Autodesk Inventor part; units mm, degrees
ref_plane "YZ Plane" through (0, 0, 0) normal (1, 0, 0) x (0, 1, 0)
ref_plane "XZ Plane" through (0, 0, 0) normal (0, 1, 0) x (-1, 0, 0)
ref_plane "XY Plane" through (0, 0, 0) normal (0, 0, 1) x (1, 0, 0)
sketch "Skizze1" plane through (0, 0, 0) normal (0, 1, 0) x (-1, 0, 0)
  circle A0 centre (0, 0) radius 31.25
  circle A1 centre (0, 0) radius 33
  line L0 (0, 109.2005) -> (0, -98.3382) construction
  line L1 (65.6021, 0) -> (-69.7309, 0) construction
  line L2 (-37.5074, 64.9647) -> (55.9703, -96.9435) construction
  line L3 (-38.0847, -65.9646) -> (43.9559, 76.1338) construction
  line L4 (30, 1.25) -> (87, 1.25)
  line L5 (87, 1.25) -> (87, -1.25)
  line L6 (87, -1.25) -> (30, -1.25)
  line L7 (30, -1.25) -> (30, 1.25)
  line L8 (28, -3.25) -> (89, -3.25)
  line L9 (89, -3.25) -> (89, 3.25)
  line L10 (89, 3.25) -> (28, 3.25)
  line L11 (28, 3.25) -> (28, -3.25)
  line L12 (-16.0825, 25.3558) -> (-44.5825, 74.7192)
  line L13 (-42.4175, 75.9692) -> (-13.9175, 26.6058)
  line L14 (-11.1854, 25.8737) -> (-41.6854, 78.7013)
  line L15 (-47.3146, 75.4513) -> (-16.8146, 22.6237)
  line L16 (-44.5825, 74.7192) -> (-42.4175, 75.9692)
  line L17 (-41.6854, 78.7013) -> (-47.3146, 75.4513)
  line L18 (-13.9175, 26.6058) -> (-16.0825, 25.3558)
  line L19 (-16.8146, 22.6237) -> (-11.1854, 25.8737)
  line L20 (-13.9175, -26.6058) -> (-42.4175, -75.9692)
  line L21 (-44.5825, -74.7192) -> (-16.0825, -25.3558)
  line L22 (-16.8146, -22.6237) -> (-47.3146, -75.4513)
  line L23 (-41.6854, -78.7013) -> (-11.1854, -25.8737)
  line L24 (-42.4175, -75.9692) -> (-44.5825, -74.7192)
  line L25 (-47.3146, -75.4513) -> (-41.6854, -78.7013)
  line L26 (-16.0825, -25.3558) -> (-13.9175, -26.6058)
  line L27 (-11.1854, -25.8737) -> (-16.8146, -22.6237)
  point P0 (-32.8011, 56.8131)
  point P1 (-32.8011, -56.8131)
  point P2 (32.8396, -3.25)
  point P3 (32.8396, 3.25)
  point P4 (-13.6052, 30.0649)
  point P5 (-19.2344, 26.8149)
  point P6 (-19.2344, -26.8149)
  point P7 (-13.6052, -30.0649)
  point P8 (31.225, -1.25)
  point P9 (-14.53, -27.6666)
  point P10 (-16.695, -26.4166)
  point P11 (-16.695, 26.4166)
  point P12 (-14.53, 27.6666)
  point P13 (31.225, 1.25)
  dimension "d0" = 62.5
  dimension "d1" = 66
  dimension "d2" = 120
  dimension "d3" = 120
  dimension "d4" = 2.5
  dimension "d5" = 2
  dimension "d6" = 57
  dimension "d7" = 30
  dimension "d10" = 360
extrude "Extrusion1" add sketch "Skizze1" along normal blind 10 contours A0 L10 A1 L4 | L6 A1 L8 A0 | A0 L14 A1 L10 | A1 L10 L9 L8 L6 L5 L4 | L8 A1 L23 A0 | A0 L13 A1 L14 | L23 A1 L20 A0 | A1 L13 L16 L12 L15 L17 L14 | L23 L25 L22 A1 L21 L24 L20 | A0 L15 A1 L12 | L21 A1 L22 A0 | A0 L22 A1 L15
fillet "Rundung1" radius 2 6 edges at (-31.225, 5, -1.25) (-31.225, 5, 1.25) (14.53, 5, 27.6666) (16.695, 5, 26.4166) (16.695, 5, -26.4166) (14.53, 5, -27.6666)
chamfer "Fase1" distance 1 angle 45 15 edges at (-15.625, 10, -27.0633) (14.3424, 10, -28.3783) (28.9402, 10, -52.6258) (-31.7475, 10, -1.7683) (-60.0454, 10, -1.25) (31.25, 10, 0) (17.4051, 10, 26.61) (31.1052, 10, 51.3758) (17.4051, 10, -26.61) (31.1052, 10, -51.3758) (-15.625, 10, 27.0633) (-31.7475, 10, 1.7683) (-60.0454, 10, 1.25) (14.3424, 10, 28.3783) (28.9402, 10, 52.6258)
sketch "Skizze2" plane through (0, 0, 0) normal (0, 1, 0) x (-1, 0, 0)
  line L0 (-47.3146, 75.4513) -> (-19.2344, 26.8149)
  line L1 (-38.5127, 60.2059) -> (-38.5127, -59.496)
  line L2 (-38.5127, -59.496) -> (-38.5127, -60.2059)
  line L3 (-19.2344, -26.8149) -> (-47.3146, -75.4513)
  line L4 (-42.8652, 67.7448) -> (-42.8652, -67.7448)
  line L5 (-42.8652, -59.496) -> (-42.8652, -60.2059)
  line L6 (-38.5127, 60.2059) -> (-42.8652, 67.7448)
  line L7 (-38.4567, -60.109) -> (-42.8652, -67.7448)
  line L8 (-32.8835, -63.4559) -> (70.7814, -3.605)
  line L9 (70.7814, -3.605) -> (71.3962, -3.25)
  line L10 (-37.2361, -70.9948) -> (80.1013, -3.25)
  line L11 (72.9577, -7.3744) -> (73.5725, -7.0194)
  line L12 (-32.8835, -63.4559) -> (-37.2361, -70.9948)
  line L13 (71.2843, -3.25) -> (80.1013, -3.25)
  line L14 (71.3962, 3.25) -> (-32.2687, 63.101)
  line L15 (-32.2687, 63.101) -> (-32.8835, 63.4559)
  line L16 (80.1013, 3.25) -> (-37.2361, 70.9948)
  line L17 (-30.0925, 66.8704) -> (-30.7073, 67.2254)
  line L18 (71.3962, 3.25) -> (80.1013, 3.25)
  line L19 (-32.8276, 63.359) -> (-37.2361, 70.9948)
  point P0 (0, 0)
  point P1 (-41.6854, -78.7013)
  point P2 (-13.6052, -30.0649)
  point P3 (32.8396, -3.25)
  point P4 (89, -3.25)
  point P5 (89, 3.25)
  point P6 (32.8396, 3.25)
  point P7 (-13.6052, 30.0649)
  point P8 (-41.6854, 78.7013)
  dimension "d20" = 360
extrude "Extrusion2" add sketch "Skizze2" along normal blind 10
properties part number "_3D-Druck"
Model file for the job. Use its own axes, mm. A direction names the side the tool comes from. Coordinates: 2 decimals unless noted, no trailing zeros. Loops run counter-clockwise (first coordinate to the right, second up) from the corner with the lowest first, then second, coordinate; pieces in that order, holes last. Notation, with made-up numbers: M -17.75,55 L 14.25,55 A19 cw 14.25,80 Z; hole C 39,-34.5 d5. An arc over 180 degrees is marked long. Use CSV: the item, a comma, the result in double quotes. Start each with the question number.
1. Band-saw the part on A-A, the plane z = 48. List the corners of the cut face in (x, y), then the cut area to 3 significant figures.
2. Band-saw the part on B-B, the plane x = -35. List the corners of the cut face in (y, z), then the cut area to 3 significant figures.
3. Two-plate mould, pull along X, no slides. Class faces 5 (the flat face through (-85, 5, 3.25)), 6 (the flat face through (23.11, 4.93, 46.53)), 7 (the flat face through (-89, 5, 0)): pulls with the +X half, pulls with the -X half, needs draft (parallel to the pull), parting line crosses it, or undercut.
4. Flat gauge pins, fed straight in: pin 1 (4.5 mm diameter, centred on x = -67, y = 3.5, fed in from +Z); pin 2 (4 mm diameter, centred on y = 1, z = -35, fed in from -X); pin 3 (1.5 mm diameter, centred on x = 25, z = 14.5, fed in from -Y); pin 4 (2.5 mm diameter, centred on x = -86, y = 7, fed in from -Z). Where does each tip first touch, or does it go through?
5. Band-saw the part on C-C, the plane y = 7. Give the number of separate pieces and of enclosed holes in the cut face, then the cut area to 3 significant figures.
6. Probe probe 1 along X at (y, z) = (2.75, 37); probe 2 along Z at (x, y) = (-21, 3.5); probe 3 along X at (y, z) = (6.75, -7). List the from-to ranges inside material, lowest first. Write a range as [from, to].
7. Tool access for faces 1 (the cylindrical face through (-15.26, 4.44, 27.27)), 2 (the flat face through (44.539, 4.93, -77.054)), 3 (the flat face through (28.325, 9.493, -52.546)), 4 (the flat face through (45.059, 4.93, -71.544)): list every direction of +Z, -Z, +X, -X, +Y, -Y with a clear straight run to the whole face (end or side of a thin tool).
Entries:
1,outline,"M -2.59,0 L 6.11,0 L 6.11,10 L -2.59,10 Z; M 23.96,0 L 26.27,0 L 26.27,9 L 25.11,10 L 23.96,10 Z; M 29.16,0 L 31.47,0 L 31.47,10 L 30.31,10 L 29.16,9 Z; M 38.51,0 L 42.87,0 L 42.87,10 L 38.51,10 Z"
1,area,"176 mm2"
2,outline,"M 0,-29.29 L 10,-29.29 L 10,-24.26 L 0,-24.26 Z; M 0,-3.25 L 10,-3.25 L 10,-2.25 L 9,-1.25 L 0,-1.25 Z; M 0,1.25 L 9,1.25 L 10,2.25 L 10,3.25 L 0,3.25 Z; M 0,24.26 L 10,24.26 L 10,29.29 L 0,29.29 Z"
2,area,"140 mm2"
3,face 5,"needs draft"
3,face 6,"undercut"
3,face 7,"pulls with the -X half"
4,pin 1,"stops at z = 12.11"
4,pin 2,"stops at x = -28.57"
4,pin 3,"passes through"
4,pin 4,"stops at z = -3.25"
5,separate pieces,"1"
5,enclosed holes,"4"
5,area,"2,690 mm2"
6,probe 1,"x = [-21.64, -12.94], [17.61, 19.92], [22.81, 25.11], [38.51, 42.87]"
6,probe 2,"z = [-37.37, -32.35], [-25.46, -23.14], [23.14, 25.46], [32.35, 37.37]"
6,probe 3,"x = [-73.61, -64.9], [-32.25, -30.46], [30.46, 32.25], [38.51, 42.87]"
7,face 1,"+Y, -Y"
7,face 2,"-Z, +X, +Y, -Y"
7,face 3,"+Y"
7,face 4,"+X, +Y, -Y"
